Check sheet for the drawn part. Datum: minimum x, y, z corner. Units: mm. Round coordinates to 2 decimals unless told otherwise and drop trailing zeros. Order: outer loops, then holes, each group sorted by start corner. A loop starts at its lowest first (then second) coordinate and runs counter-clockwise, first axis right, second up.
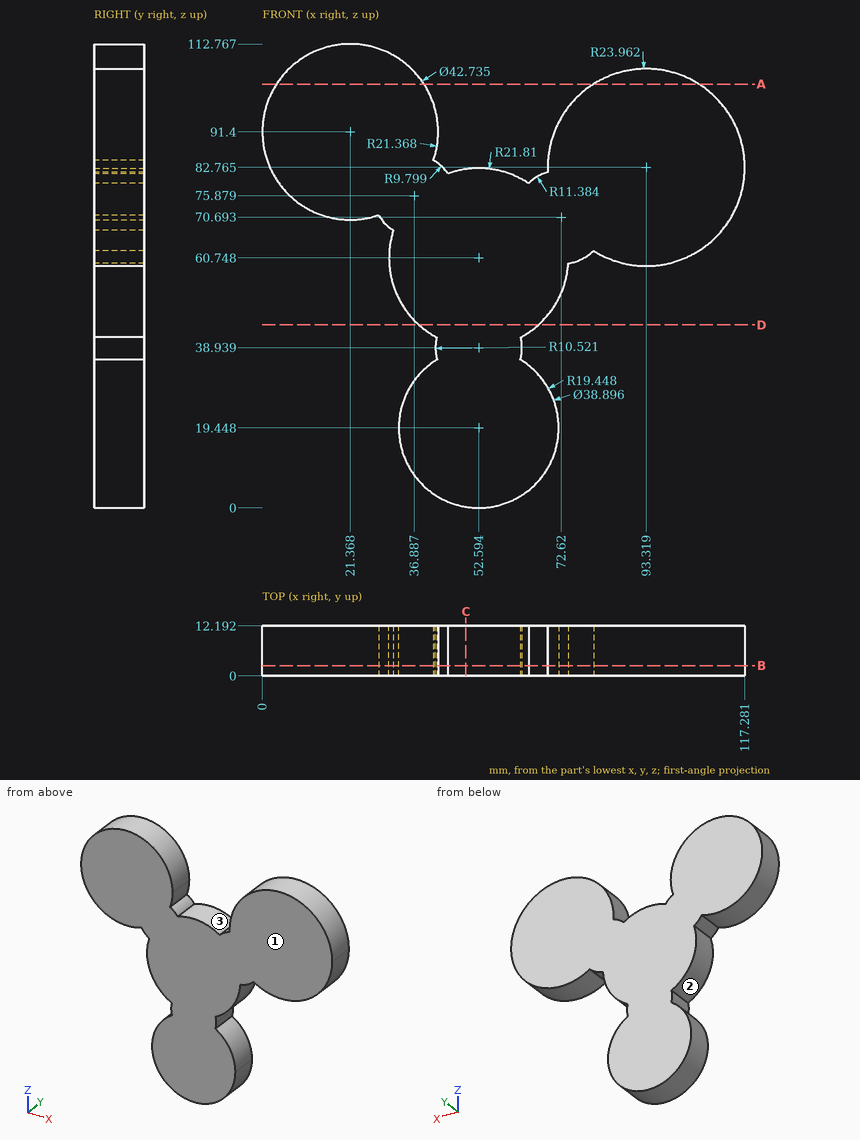
(1) Material ranges on line 1 (Z direction, x = 92.5, y = 4.5); line 2 (X direction, y = 2.5, z = 102) (1 decimal); line 3 (X direction, y = 7, z = 79.5) (1 decimal), recorded low to high.
Returned:
line 1: z = 58.82 to 106.71
line 2: x = 2.8 to 39.9, 79 to 107.6
line 3: x = 3.6 to 63.7, 65.4 to 117.1
(2) Depth check by flat-ended pin: P1, Ø3, axis at x = 32, y = 8, coming from the +Z side; P2, Ø4, axis at x = 13.5, y = 10.5, coming from the -Z side; P3, Ø3, axis at y = 1.5, z = 68, coming from the +X side (1 decimal). Enter the tip coordinate at first touch or a pass-through.
Returned:
P1: stops at z = 110.72
P2: stops at z = 70.85
P3: stops at x = 113.3
(3) Draft check along X on the marked faces 1, 2 and 3. Enter one of: released by +X, released by -X, zero draft, split by the parting line, or undercut.
Returned:
face 1: zero draft
face 2: released by -X
face 3: undercut
(4) Sectioned sample at B-B, the plane y = 2.5. Record the cut outline in (x, z) (1 decimal).
Returned:
outline: (28.3, 71.2) arc R9.8 ccw to (31.8, 67.5) arc R21.8 ccw to (42.4, 41.5) arc R10.5 ccw to (42.5, 36.1) arc R19.4 ccw (long way) to (62.7, 36.1) arc R10.5 ccw to (62.8, 41.5) arc R21.8 ccw to (74.4, 59.4) arc R11.4 ccw to (80.5, 62.5) arc R24 ccw (long way) to (69.4, 81.6) arc R11.4 ccw to (64.7, 78.9) arc R21.8 ccw to (45.1, 81.2) arc R9.8 ccw to (41.6, 84.5) arc R21.4 ccw (long way) to start
(5) Sectioned sample at D-D, the plane z = 44.5. Record the cut outline in (x, y), and give its area (3 significant figures).
Returned:
outline: (38.05, 0) - (67.14, 0) - (67.14, 12.19) - (38.05, 12.19) - close
area: 355 mm2
(6) Sectioned sample at C-C, the plane x = 49.5. Record the cut outline in (y, z), and give its area (3 significant figures).
Returned:
outline: (0, 0.25) - (12.19, 0.25) - (12.19, 82.34) - (0, 82.34) - close
area: 1,000 mm2
(7) Sectioned sample at A-A, the plane z = 103. Record the cut outline in (x, y) (1 decimal).
Returned:
outline: (3.4, 0) - (39.3, 0) - (39.3, 12.2) - (3.4, 12.2) - close; (80.5, 0) - (106.2, 0) - (106.2, 12.2) - (80.5, 12.2) - close
